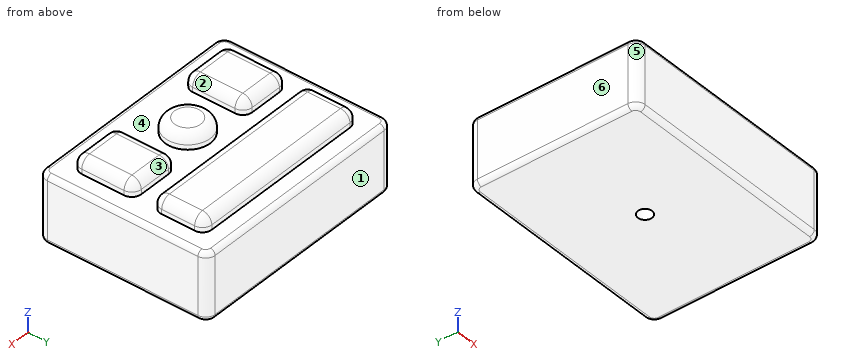
from build123d import *

# Parameters (mm, degrees)
F0_W     = 238
F0_H     = 180
F1_DEPTH = 86
F2_W     = 238
F2_H     = 180
F2_W_2   = 55
F2_H_2   = 65
F2_R     = 24
F2_W_3   = 198
F2_H_3   = 55
F3_DEPTH = 15
F4_R     = 10
F5_R     = 10
F6_R     = 5
F7_R     = 7.5
F8_DEPTH = 50


with BuildPart() as f1:
    # F0 (on Top) → F1 (new body)
    with BuildSketch(Plane.XY):
        Rectangle(F0_W, F0_H)
    extrude(amount=F1_DEPTH)

    # F2 (on face) → F3 (cut)
    with BuildSketch(Plane.XY.offset(86)):
        Rectangle(F2_W, F2_H)
        with Locations((-71.5, -37.5)):
            Rectangle(F2_W_2, F2_H_2, mode=Mode.SUBTRACT)
        with Locations((0, -29)):
            Circle(F2_R, mode=Mode.SUBTRACT)
        with Locations((71.5, -37.5)):
            Rectangle(F2_W_2, F2_H_2, mode=Mode.SUBTRACT)
        with Locations((0, 42.5)):
            Rectangle(F2_W_3, F2_H_3, mode=Mode.SUBTRACT)
    extrude(amount=-F3_DEPTH, mode=Mode.SUBTRACT)

    # F4
    f4_edges = [f1.edges().sort_by_distance(p)[0] for p in [
        (-119, -90, 35.5),
        (119, -90, 35.5),
        (-119, 90, 35.5),
        (119, 90, 35.5),
        (-99, 70, 78.5),
        (-99, -5, 78.5),
        (-99, -70, 78.5),
        (-44, -5, 78.5),
        (99, 70, 78.5),
        (99, -5, 78.5),
        (44, -5, 78.5),
        (44, -70, 78.5),
        (-99, 15, 78.5),
        (-44, -70, 78.5),
        (99, -70, 78.5),
        (99, 15, 78.5),
    ]]
    fillet(f4_edges, radius=F4_R)

    # F5
    f5_edges = [f1.edges().sort_by_distance(p)[0] for p in [
        (0, 15, 86),
        (-71.5, -5, 86),
        (-24, -29, 86),
        (71.5, -5, 86),
    ]]
    fillet(f5_edges, radius=F5_R)

    # F6
    f6_edges = [f1.edges().sort_by_distance(p)[0] for p in [
        (-119, 0, 71),
        (-119, 0, 0),
    ]]
    fillet(f6_edges, radius=F6_R)

    # F7 (on face) → F8 (cut)
    with BuildSketch(Plane(origin=(0, 0, 0), x_dir=(1, 0, 0), z_dir=(0, 0, -1))):
        Circle(F7_R)
    extrude(amount=-F8_DEPTH, mode=Mode.SUBTRACT)


solid = f1.part
The model under review builds one solid part; all positions refer to its coordinate system, in mm. Face numbers are marked on the shaded views. A direction names the side the tool comes from. Round coordinates to 2 decimals unless told otherwise and drop trailing zeros. Write each loop counter-clockwise with the first axis right and the second up, starting at its lowest first coordinate (ties: lowest second). Pieces come first, ordered by that corner, then holes. Notation, with made-up numbers: M -25,23.25 L -1,23.25 A26 cw -1,48.25 Z; hole C 26.5,15.5 d8. An arc over 180 degrees is marked long. Use a Markdown table: item, result. Add a question column.
Q1. The part is to be moulded in two halves that separate along Y. For the marked faces 4, 5 and 6, say which applies: pulls with the +Y half, pulls with the -Y half, needs draft (parallel to the pull), parting line crosses it, or undercut.
Q2. We need section D-D, the plane y = 0. State the section outline as (x, z) points.
Q3. We need section B-B, the plane y = -29. State the section outline as (x, z) points.
Q4. Machinability: for the marked faces 1, 2 and 3, which of the approach directions +Z, -Z, +X, -X, +Y, -Y give a long, thin tool a straight path to every point of the face, cutting with its end or side? Answer none if there is none.
Q5. Insertion check: pin 1 (2.5 mm diameter, centred on x = 79, z = 72.5, fed in from +Y); pin 2 (1.5 mm diameter, centred on x = 7, z = 74.5, fed in from -Y); pin 3 (5 mm diameter, centred on y = -3, z = 70, fed in from -X). Each pin has a flat end and moves straight along its axis. Give the tip position at first contact, or say it passes through.
Q6. We need section C-C, the plane x = -31.5. State the section outline as (y, z) points.
Q7. To check wall thickness, follow line 1 (Y direction, x = 0, z = 15); line 2 (X direction, y = 0, z = 39.5); line 3 (Y direction, x = 28, z = 75). State the ranges of each line that lie inside material, in increasing order.
Q8. We need section A-A, the plane x = -77. State the section outline as (y, z) points, plus the area to 3 significant figures.
Findings below:
| question | item | result |
|---|---|---|
| 1 | face 4 | undercut |
| 1 | face 5 | pulls with the -Y half |
| 1 | face 6 | needs draft |
| 2 | outline | M -119,5 A5 ccw -114,0 L -7.5,0 L -7.5,50 L 7.5,50 L 7.5,0 L 114,0 A5 ccw 119,5 L 119,66 A5 ccw 114,71 L -114,71 A5 ccw -119,66 Z |
| 3 | outline | M -119,5 A5 ccw -114,0 L 114,0 A5 ccw 119,5 L 119,66 A5 ccw 114,71 L 99,71 L 99,76 A10 ccw 89,86 L 54,86 A10 ccw 44,76 L 44,71 L 24,71 L 24,76 A10 ccw 14,86 L -14,86 A10 ccw -24,76 L -24,71 L -44,71 L -44,76 A10 ccw -54,86 L -89,86 A10 ccw -99,76 L -99,71 L -114,71 A5 ccw -119,66 Z |
| 4 | face 1 | +Z, -Z, +X, -X, +Y |
| 4 | face 2 | +Z, -Y |
| 4 | face 3 | +Z, +X, -X |
| 5 | pin 1 | stops at y = 70 |
| 5 | pin 2 | stops at y = -52.17 |
| 5 | pin 3 | stops at x = -118.77 |
| 6 | outline | M -90,5 A5 ccw -85,0 L 85,0 A5 ccw 90,5 L 90,66 A5 ccw 85,71 L 70,71 L 70,76 A10 ccw 60,86 L 25,86 A10 ccw 15,76 L 15,71 L -85,71 A5 ccw -90,66 Z |
| 7 | line 1 | y = -90 to -7.5, 7.5 to 90 |
| 7 | line 2 | x = -119 to -7.5, 7.5 to 119 |
| 7 | line 3 | y = 15 to 70 |
| 8 | outline | M -90,5 A5 ccw -85,0 L 85,0 A5 ccw 90,5 L 90,66 A5 ccw 85,71 L 70,71 L 70,76 A10 ccw 60,86 L 25,86 A10 ccw 15,76 L 15,71 L -5,71 L -5,76 A10 ccw -15,86 L -60,86 A10 ccw -70,76 L -70,71 L -85,71 A5 ccw -90,66 Z |
| 8 | area | 14,500 mm² |
